Autodesk Inventor part; units mm, degrees
ref_plane "YZ Plane" through (0, 0, 0) normal (1, 0, 0) x (0, 1, 0)
ref_plane "XZ Plane" through (0, 0, 0) normal (0, 1, 0) x (-1, 0, 0)
ref_plane "XY Plane" through (0, 0, 0) normal (0, 0, 1) x (1, 0, 0)
sketch "Sketch1" plane through (0, 0, 0) normal (0, 0, 1) x (1, 0, 0)
  line L0 (0, 0) -> (42, 0)
  line L1 (42, 0) -> (42, 29)
  line L2 (42, 29) -> (0, 29)
  line L3 (0, 29) -> (0, 0)
  dimension "d0" = 42
  dimension "d1" = 29
extrude "Extrusion1" add sketch "Sketch1" along normal blind 29
sketch "Sketch2" plane through (42, 0, 0) normal (1, 0, 0) x (0, 0, -1)
  line L0 (0, 0) -> (0, 29)
  line L1 (0, 29) -> (-29, 29)
  line L2 (-29, 0) -> (-29, 29)
  line L3 (0, 0) -> (-29, 0)
  circle A0 centre (-14.5, 14.5) radius 14.2
  circle A1 centre (-14.5, 14.5) radius 12.7369
  dimension "d4" = 28.4
extrude "Extrusion2" add sketch "Sketch2" along normal blind 12 contours A0
sketch "Sketch3" plane through (0, 0, 0) normal (-1, 0, 0) x (0, 0, 1)
  line L0 (0, 29) -> (0, 0)
  line L1 (0, 0) -> (29, 0)
  line L2 (29, 29) -> (29, 0)
  line L3 (0, 29) -> (29, 29)
  circle A0 centre (14.5, 14.5) radius 14.2
  circle A1 centre (4.4212, 4.4971) radius 4
  dimension "d7" = 8
extrude "Extrusion3" add sketch "Sketch3" along normal blind 8 contours A1 A0 | A0 A1 picked at (5.4383, 5.4228) picked at (3.5046, 3.5874)
sketch "Sketch4" plane through (0, 0, 0) normal (0, -1, 0) x (1, 0, 0)
  line L0 (0, 0) -> (42, 0)
  line L1 (42, 0) -> (42, 29)
  line L2 (0, 29) -> (42, 29)
  line L3 (0, 0) -> (0, 29)
  line L4 (54, 0.3) -> (54, 28.7)
  line L5 (42, 28.7) -> (42, 0.3)
  line L6 (54, 14.5) -> (0, 14.5) construction
  line L7 (0, 0) -> (0, 29) construction
  point P0 (38.8, 4.5)
  point P1 (38.8, 24.5)
  point P2 (15.3, 14.5)
  dimension "d10" = 10
  dimension "d11" = 14.5
  dimension "d12" = 3.2
  dimension "d13" = 10
  dimension "d14" = 3.2
  dimension "d15" = 23.5
hole "Hole1" at (38.8, 0, 4.5) at (38.8, 0, 24.5) at (15.3, 0, 14.5) direction (0, 1, 0) diameter 2.8 depth 12 tip angle 118
properties part number "00_Basler_acA1920_25gm"
Can you work these out from the model? Positions are in its coordinate system, mm. A direction names the side the tool comes from. Give positions to 0.01 mm unless a question says otherwise; leave off trailing zeros. Loops run counter-clockwise (first coordinate to the right, second up) from the corner with the lowest first, then second, coordinate; pieces in that order, holes last. Notation, with made-up numbers: M 42.5,18 L 101.5,18 A21 ccw 101.5,46 Z; hole C 20.5,28 d3. An arc over 180 degrees is marked long. Answer in a Markdown table with one row per item.
1. For pin 1 Ø8 at (y, z) = (17.5, 14.5) entering from -X; pin 2 Ø4 at (x, y) = (46, 14.5) entering from -Z; pin 3 Ø14.5 at (y, z) = (13, 11) entering from +X, each with a flat end and sliding along its axis, tell me the tip position at first contact or that it passes through.
Taken from the geometry:
| item | result |
|---|---|
| pin 1 | stops at x = 0 |
| pin 2 | stops at z = 0.3 |
| pin 3 | stops at x = 42 |
2. Suppose I cut it at D-D on y = 19.5. Write out the boundary of the cut face in (x, z), plus the area to 3 significant figures.
Taken from the geometry:
| item | result |
|---|---|
| outline | M 0,0 L 42,0 L 42,1.21 L 54,1.21 L 54,2.79 L 42,2.79 L 42,26.21 L 54,26.21 L 54,27.79 L 42,27.79 L 42,29 L 0,29 Z |
| area | 1,260 mm² |
3. Suppose I cut it at A-A on z = 2.5. Write out the boundary of the cut face in (x, y).
Taken from the geometry:
| item | result |
|---|---|
| outline | M -8,0.99 L 0,0.99 L 0,0 L 42,0 L 42,6.91 L 54,6.91 L 54,10.23 L 42,10.23 L 42,18.77 L 54,18.77 L 54,22.09 L 42,22.09 L 42,29 L 0,29 L 0,8.01 L -8,8.01 Z |
4. If I drill on line 1 along Z through (x, y) = (38.8, 7.75); line 2 along X through (y, z) = (6.25, 4.5); line 3 along Y through (x, z) = (45.5, 14.5), over which ranges is the centre line in solid material (lowest first)?
Taken from the geometry:
| item | result |
|---|---|
| line 1 | z = 0 to 3.1, 5.9 to 23.1, 25.9 to 29 |
| line 2 | x = -8 to 37.4, 40.2 to 54 |
| line 3 | y = 0.3 to 1.76, 27.24 to 28.7 |
5. Which directions (+Z, -Z, +X, -X, +Y, -Y) give clear straight access to the entire face, cutting with the end or side of a thin tool? Please do faces 4 (the cylindrical face through (47.92, 22.25, 24.61)), 5 (the cylindrical face through (39.34, 6.08, 23.21)), 6 (the cylindrical face through (-3.94, 8.4, 3.55)).
Taken from the geometry:
| item | result |
|---|---|
| face 4 | +X |
| face 5 | -Y |
| face 6 | -X |
6. Suppose I cut it at C-C on x = 44.5. Write out the boundary of the cut face in (y, z).
Taken from the geometry:
| item | result |
|---|---|
| outline | C 14.5,14.5 d28.4; hole C 14.5,14.5 d25.47 |
7. Suppose I cut it at B-B on y = 10.25. Write out the boundary of the cut face in (x, z).
Taken from the geometry:
| item | result |
|---|---|
| outline | M 0,0 L 42,0 L 42,0.95 L 54,0.95 L 54,2.49 L 42,2.49 L 42,26.51 L 54,26.51 L 54,28.05 L 42,28.05 L 42,29 L 0,29 Z; hole C 15.3,14.5 d2.8; hole C 38.8,4.5 d2.8; hole C 38.8,24.5 d2.8 |
8. Thinking about a two-plate mould opening in X: for faces 1 (the flat face through (21, 15, 0)), 2 (the cylindrical face through (39.34, 6.08, 3.21)), 3 (the flat face through (42, 1.5, 8)), which applies, released by +X, released by -X, zero draft, split by the parting line, or undercut?
Taken from the geometry:
| item | result |
|---|---|
| face 1 | zero draft |
| face 2 | undercut |
| face 3 | released by +X |
